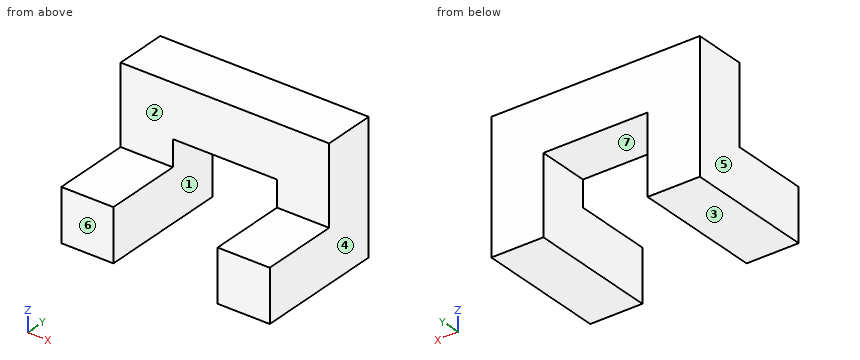
```python
from build123d import *

# Parameters (mm, degrees)
F1_DEPTH = 50.8
F2_W     = 50.8
F2_H     = 50.8
F3_DEPTH = 76.2
F4_W     = 50.8
F4_H     = 50.8
F5_DEPTH = 76.2


with BuildPart() as f1:
    # F0 (on Front) → F1 (new body)
    with BuildSketch(Plane.XZ):
        Polygon((-72.271809, 79.84082), (-72.271809, -47.15918), (-21.471809, -47.15918), (-21.471809, 29.04082), (80.128191, 29.04082), (80.128191, -47.15918), (130.928191, -47.15918), (130.928191, 79.84082), align=None)
    extrude(amount=F1_DEPTH)

    # F2 (on face) → F3 (join)
    with BuildSketch(Plane.XZ.offset(50.8)):
        with Locations((-46.871809, -21.75918)):
            Rectangle(F2_W, F2_H)
    extrude(amount=F3_DEPTH)

    # F4 (on face) → F5 (join)
    with BuildSketch(Plane.XZ.offset(50.8)):
        with Locations((105.528191, -21.75918)):
            Rectangle(F4_W, F4_H)
    extrude(amount=F5_DEPTH)


solid = f1.part
```
Geometry: final body of the model. Coordinates: model frame, mm. Face numbers are marked on the shaded views. A direction names the side the tool comes from. Round coordinates to 2 decimals unless told otherwise and drop trailing zeros. Write each loop counter-clockwise with the first axis right and the second up, starting at its lowest first coordinate (ties: lowest second). Pieces come first, ordered by that corner, then holes. Notation, with made-up numbers: (-6.75, 38) -> (29.25, 38) arc R31 ccw to (29.25, 65) -> close; hole circle Ø4 at (-9, 47.25). An arc over 180 degrees is marked (long way). Use CSV: the item, a comma, the result in double quotes. Start each with the question number.
Q1. Section C-C (y = -8.5). Return loops of the section in (x, z).
Q2. Section B-B (z = -6). Return loops of the section in (x, y).
Q3. Line query: L1, parallel to X at y = -15, z = -25; L2, parallel to Y at x = 109, z = 35; L3, parallel to Z at x = 66.5, y = -25. Output: solid intervals per line, ascending.
Q4. First-contact query: pin 1 Ø15 at (x, y) = (47, -29.5) entering from -Z; pin 2 Ø8 at (x, y) = (76, -82.5) entering from -Z. Flat tips, straight axial feed; report the tip coordinate or a pass-through.
Q5. Section A-A (y = -111). Return loops of the section in (x, z).
Q6. Section D-D (x = 90). Return loops of the section in (y, z).
Q7. Reachability of the marked faces 1, 2 and 3 from +Z, -Z, +X, -X, +Y, -Y: full face, straight path, thin tool, end or side. Return the list, or none.
Q8. Pull-direction query (X, two-part tool) for the marked faces 4, 5, 6 and 7; classes: pulls with the +X half, pulls with the -X half, needs draft (parallel to the pull), parting line crosses it, or undercut.
Result sheet:
1,outline,"(-72.27, -47.16) -> (-21.47, -47.16) -> (-21.47, 29.04) -> (80.13, 29.04) -> (80.13, -47.16) -> (130.93, -47.16) -> (130.93, 79.84) -> (-72.27, 79.84) -> close"
2,outline,"(-72.27, -127) -> (-21.47, -127) -> (-21.47, 0) -> (-72.27, 0) -> close; (80.13, -127) -> (130.93, -127) -> (130.93, 0) -> (80.13, 0) -> close"
3,L1,"-72.27 to -21.47, 80.13 to 130.93"
3,L2,"-50.8 to 0"
3,L3,"29.04 to 79.84"
4,pin 1,"z = 29.04"
4,pin 2,"through"
5,outline,"(-72.27, -47.16) -> (-21.47, -47.16) -> (-21.47, 3.64) -> (-72.27, 3.64) -> close; (80.13, -47.16) -> (130.93, -47.16) -> (130.93, 3.64) -> (80.13, 3.64) -> close"
6,outline,"(-127, -47.16) -> (0, -47.16) -> (0, 79.84) -> (-50.8, 79.84) -> (-50.8, 3.64) -> (-127, 3.64) -> close"
7,face 1,"-Z, +Y, -Y"
7,face 2,"+Z, +X, -X, -Y"
7,face 3,"-Z, +X, -X, +Y, -Y"
8,face 4,"pulls with the +X half"
8,face 5,"pulls with the -X half"
8,face 6,"needs draft"
8,face 7,"undercut"
